Geometry: see drawing. Coordinates: mm, zero at the bounding-box minimum. A direction names the side the tool comes from. Coordinates: 2 decimals unless noted, no trailing zeros. Order: outer loops, then holes, each group sorted by start corner. A loop starts at its lowest first (then second) coordinate and runs counter-clockwise, first axis right, second up. Notation, with made-up numbers: M 78.5,73.25 L 102.5,73.25 A18 cw 102.5,81.25 Z; hole C -7.5,5 d6. An arc over 180 degrees is marked long. Answer in a Markdown table with one row per item.
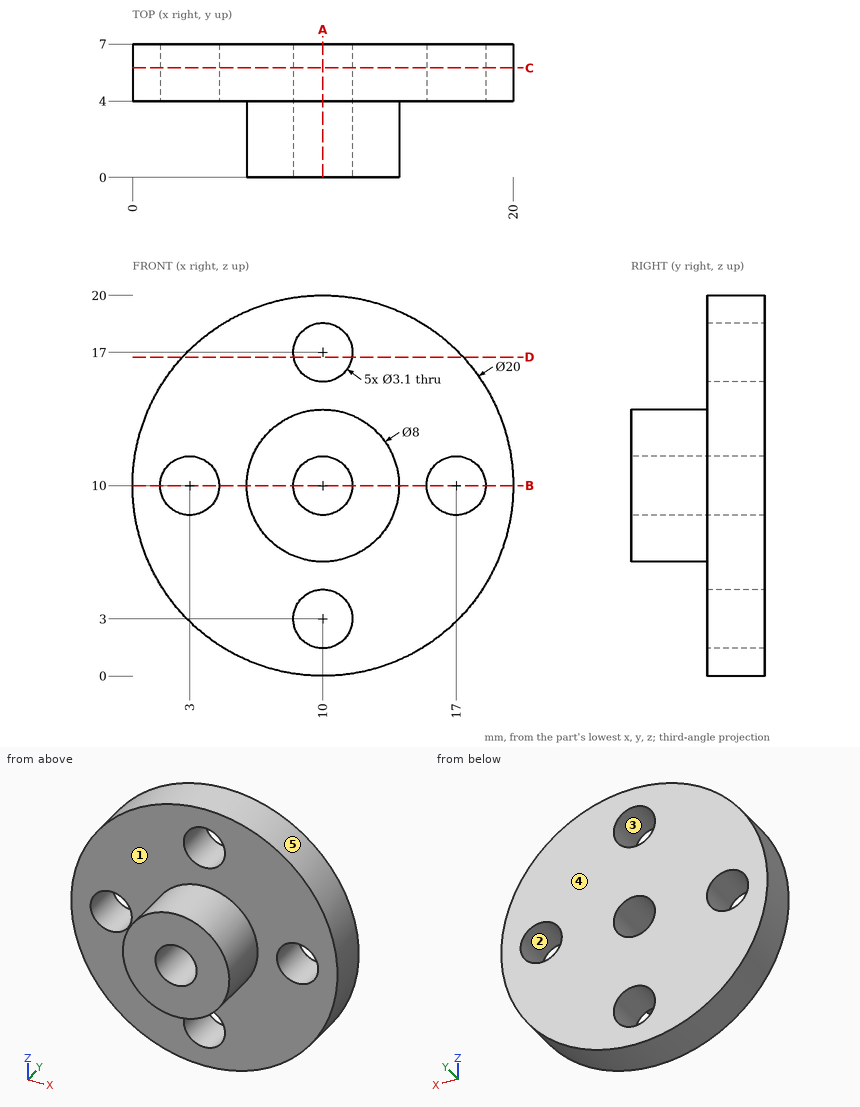
1) Material intervals for probe 1 along X at (y, z) = (5.75, 10); probe 2 along X at (y, z) = (4.25, 9); probe 3 along X at (y, z) = (2.25, 10), sorted ascending.
Resolved:
| item | result |
|---|---|
| probe 1 | x = 0 to 1.45, 4.55 to 8.45, 11.55 to 15.45, 18.55 to 20 |
| probe 2 | x = 0.05 to 1.82, 4.18 to 8.82, 11.18 to 15.82, 18.18 to 19.95 |
| probe 3 | x = 6 to 8.45, 11.55 to 14 |
2) Contact query for flat-ended pins moving along their axis: pin 1 (3 mm diameter, centred on y = 6, z = 4, fed in from -X); pin 2 (5 mm diameter, centred on x = 3, z = 10, fed in from -Y); pin 3 (3 mm diameter, centred on x = 10, z = 10, fed in from +Y); pin 4 (1 mm diameter, centred on y = 1, z = 9, fed in from +X). Output: stop coordinate, or through.
Resolved:
| item | result |
|---|---|
| pin 1 | stops at x = 1.07 |
| pin 2 | stops at y = 4 |
| pin 3 | passes through |
| pin 4 | stops at x = 13.97 |
3) Cut plane D-D, the plane z = 16.75. Output: boundary loops of the cut face in (x, y).
Resolved:
| item | result |
|---|---|
| outline | M 2.62,4 L 8.47,4 L 8.47,7 L 2.62,7 Z; M 11.53,4 L 17.38,4 L 17.38,7 L 11.53,7 Z |
4) Cut plane C-C, the plane y = 5.75. Output: boundary loops of the cut face in (x, z).
Resolved:
| item | result |
|---|---|
| outline | C 10,10 d20; hole C 3,10 d3.1; hole C 10,3 d3.1; hole C 10,10 d3.1; hole C 10,17 d3.1; hole C 17,10 d3.1 |
5) Mould query, pull axis Z, two halves, no side actions, for the marked faces 3, 4 and 5. Classes: +Z half, -Z half, draft (parallel to the pull), parting line (faces both ways), or undercut.
Resolved:
| item | result |
|---|---|
| face 3 | undercut |
| face 4 | draft |
| face 5 | parting line |
6) Reachability of the marked faces 1 and 2 from +Z, -Z, +X, -X, +Y, -Y: full face, straight path, thin tool, end or side. Return the list, or none.
Resolved:
| item | result |
|---|---|
| face 1 | -Y |
| face 2 | +Y, -Y |
7) Cut plane B-B, the plane z = 10. Output: boundary loops of the cut face in (x, y).
Resolved:
| item | result |
|---|---|
| outline | M 0,4 L 1.45,4 L 1.45,7 L 0,7 Z; M 4.55,4 L 6,4 L 6,0 L 8.45,0 L 8.45,7 L 4.55,7 Z; M 11.55,0 L 14,0 L 14,4 L 15.45,4 L 15.45,7 L 11.55,7 Z; M 18.55,4 L 20,4 L 20,7 L 18.55,7 Z |
8) Cut plane A-A, the plane x = 10. Output: boundary loops of the cut face in (y, z).
Resolved:
| item | result |
|---|---|
| outline | M 0,6 L 4,6 L 4,4.55 L 7,4.55 L 7,8.45 L 0,8.45 Z; M 0,11.55 L 7,11.55 L 7,15.45 L 4,15.45 L 4,14 L 0,14 Z; M 4,0 L 7,0 L 7,1.45 L 4,1.45 Z; M 4,18.55 L 7,18.55 L 7,20 L 4,20 Z |
